```python
from build123d import *

# Parameters (mm, degrees)
BOSS_EXTRUDE1_DEPTH = 15
SKETCH4_W           = 13.5
SKETCH4_H           = 15
BOSS_EXTRUDE2_DEPTH = 4.8
CUT_EXTRUDE1_DEPTH  = 5.5
SKETCH6_R           = 5.75
CUT_EXTRUDE2_DEPTH  = 2.2
SKETCH7_R           = 2.75
CUT_EXTRUDE3_DEPTH  = 1.8
FILLET1_R           = 1
FILLET2_R           = 0.5


with BuildPart() as part:
    # Sketch1 → Boss-Extrude1 (new body)
    with BuildSketch(Plane.XY):
        Polygon((0, -2.5), (0, 0), (-16.25, 0), (-17.5, 2.727178029), (-15.5, 7.418659671), (-17.799745903, 8.399051828), (-20.233306637, 2.690549074), (-17.85422237, -2.5), align=None)
        Polygon((17.5, 2.727178029), (16.25, 0), (0, 0), (0, -2.5), (17.85422237, -2.5), (20.233306637, 2.690549074), (17.799745903, 8.399051828), (15.5, 7.418659671), align=None)
    extrude(amount=BOSS_EXTRUDE1_DEPTH)

    # Sketch4 → Boss-Extrude2 (add)
    with BuildSketch(Plane.XZ.offset(2.5)):
        with Locations((0, 7.5)):
            Rectangle(SKETCH4_W, SKETCH4_H)
    extrude(amount=BOSS_EXTRUDE2_DEPTH)

    # Sketch5 → Cut-Extrude1 (cut)
    with BuildSketch(Plane(origin=(0, 0, 0), x_dir=(1, 0, 0), z_dir=(0, 1, 0))):
        Polygon((-4.1, -9.867136104), (0, -12.234272207), (4.1, -9.867136104), (4.1, -5.132863896), (0, -2.765727793), (-4.1, -5.132863896), align=None)
    extrude(amount=-CUT_EXTRUDE1_DEPTH, mode=Mode.SUBTRACT)

    # Sketch6 → Cut-Extrude2 (cut)
    with BuildSketch(Plane(origin=(0, 0, 0), x_dir=(1, 0, 0), z_dir=(0, 1, 0))):
        with Locations(Location((0, -7.5, 0), (0, 0, 180))):
            Circle(SKETCH6_R)
    extrude(amount=-CUT_EXTRUDE2_DEPTH, mode=Mode.SUBTRACT)

    # Sketch7 → Cut-Extrude3 (cut)
    with BuildSketch(Plane(origin=(0, -5.5, 0), x_dir=(1, 0, 0), z_dir=(0, 1, 0))):
        with Locations(Location((0, -7.5, 0), (0, 0, 180))):
            Circle(SKETCH7_R)
    extrude(amount=-CUT_EXTRUDE3_DEPTH, mode=Mode.SUBTRACT)

    # Fillet1
    fillet1_edges = [part.edges().sort_by_distance(p)[0] for p in [
        (-17.85422237, -2.5, 7.5),
        (-20.233306637, 2.690549074, 7.5),
        (20.233306637, 2.690549074, 7.5),
        (17.85422237, -2.5, 7.5),
        (-6.75, -2.5, 7.5),
        (6.75, -2.5, 7.5),
    ]]
    fillet(fillet1_edges, radius=FILLET1_R)

    # Fillet2
    fillet2_edges = [part.edges().sort_by_distance(p)[0] for p in [
        (-2.05, -2.2, 11.050704156),
        (-4.1, -2.2, 7.5),
        (-2.05, -2.2, 3.949295844),
        (2.05, -2.2, 3.949295844),
        (4.1, -2.2, 7.5),
        (2.05, -2.2, 11.050704156),
    ]]
    fillet(fillet2_edges, radius=FILLET2_R)


solid = part.part
```
Work out the finished part from the listing and answer in its coordinate system (mm). A direction names the side the tool comes from. Give positions to 0.01 mm unless a question says otherwise; leave off trailing zeros. Order: outer loops, then holes, each group sorted by start corner. A loop starts at its lowest first (then second) coordinate and runs counter-clockwise, first axis right, second up. Notation, with made-up numbers: M 78.5,89.5 L 129.5,89.5 A19 ccw 129.5,125.5 Z; hole C 48.25,71.25 d9. An arc over 180 degrees is marked long. Return JSON: item names as keys, results as strings.
1) Each of these flat-tipped pins is pushed along its axis until it touches: pin 1 (1.5 mm diameter, centred on y = -4.5, z = 11, fed in from -X); pin 2 (3 mm diameter, centred on y = -6, z = 10.5, fed in from +X); pin 3 (6 mm diameter, centred on x = 2.5, z = 8, fed in from +Y). Where does it stop, or does it pass through?
Resolved:
{"pin 1": "x = -6.75", "pin 2": "x = 6.75", "pin 3": "y = -2.2"}
2) Section A-A, the plane x = 14 is taken. Write down the section's boundary in (y, z).
Resolved:
{"outline": "M -2.5,0 L 0,0 L 0,15 L -2.5,15 Z"}
3) A tool of negligible diameter and unlimited length cuts with its end or side. For faces 5 (the flat face through (16.486, 5.106, 7.395)), 6 (the flat face through (-18.91, 5.79, 7.4)), 7 (the flat face through (4.1, -4, 8)), from which of +Z, -Z, +X, -X, +Y, -Y can it reach the whole face along a straight path? Write none if from no direction.
Resolved:
{"face 5": "+Z, -Z", "face 6": "+Z, -Z, -X, +Y", "face 7": "+Y"}
4) For a pull along X with two mould halves and no side action, classify faces 1 (the flat face through (0, -2, 0)), 2 (the flat face through (16.884, 1.383, 7.395)), 3 (the flat face through (-19, 0, 7)), 4 (the cylindrical face through (20.14, 2.69, 7.6)) as +X half, -X half, draft (parallel to the pull), parting line (faces both ways), or undercut.
Resolved:
{"face 1": "draft", "face 2": "undercut", "face 3": "-X half", "face 4": "+X half"}
5) Straight lines are drawn through the part: line 1 along Z through (x, y) = (0, -6.9); line 2 along Z through (x, y) = (0, -0.8); line 3 along Y through (x, z) = (14.5, 5). For each, find the intervals that lie inside material, in ascending order. Write a range as [from, to].
Resolved:
{"line 1": "[0, 4.75], [10.25, 15]", "line 2": "[0, 1.75], [13.25, 15]", "line 3": "[-2.5, 0]"}
